Part print with two shaded views. Sizes in mm from the minimum x, y, z corner. Round coordinates to 2 decimals unless told otherwise and drop trailing zeros. Loops run counter-clockwise (first coordinate to the right, second up) from the corner with the lowest first, then second, coordinate; pieces in that order, holes last. Notation, with made-up numbers: (85, 4.25) - (131, 4.25) arc R6 ccw to (131, 13.25) - close; hole circle Ø10 at (45.5, -26). An arc over 180 degrees is marked (long way). Use a Markdown table: item, result.
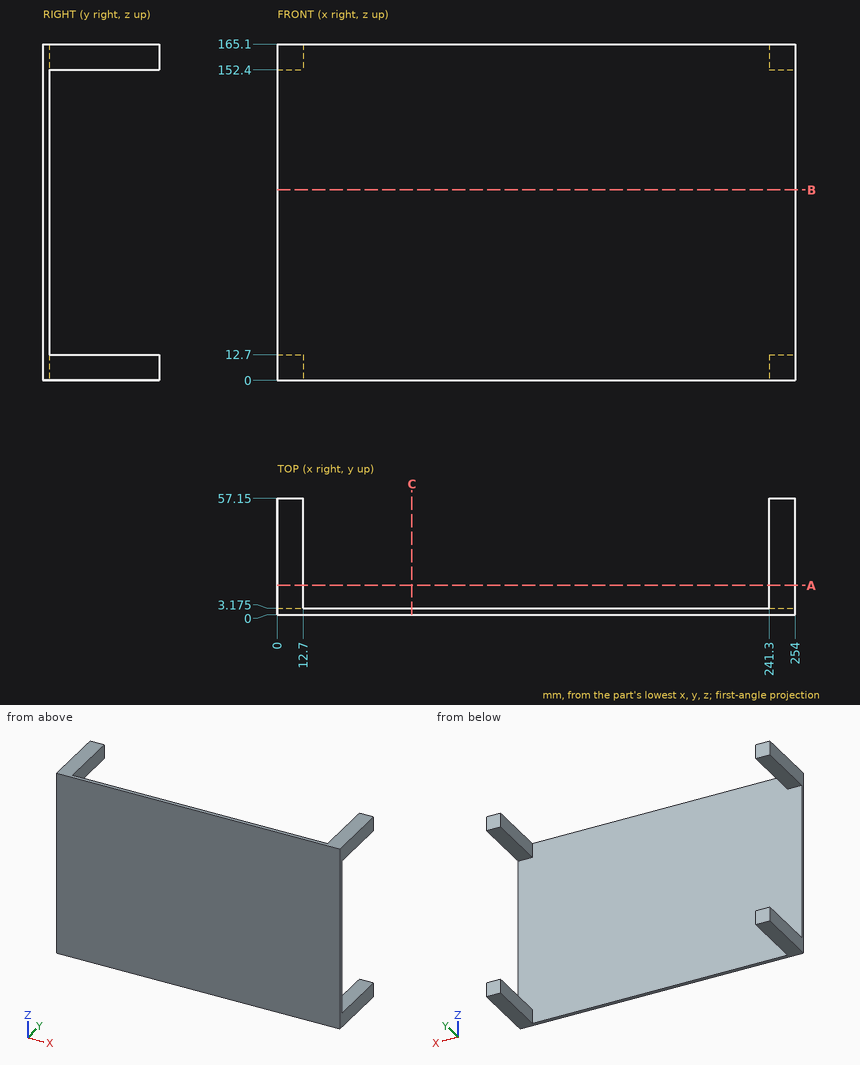
Q1. Probe line 1 (Z direction, x = 12, y = 49.5); line 2 (Y direction, x = 122.5, z = 90) (3 decimals). List the from-to ranges inside material, lowest first.
Results found:
| item | result |
|---|---|
| line 1 | z = 0 to 12.7, 152.4 to 165.1 |
| line 2 | y = 0 to 3.175 |
Q2. Cut at C-C, the plane x = 66. List the corners of the cut face in (y, z) (3 decimals), plus the area to 3 significant figures.
Results found:
| item | result |
|---|---|
| outline | (0, 0) - (3.175, 0) - (3.175, 165.1) - (0, 165.1) - close |
| area | 524 mm2 |
Q3. Cut at A-A, the plane y = 14.5. List the corners of the cut face in (x, z).
Results found:
| item | result |
|---|---|
| outline | (0, 0) - (12.7, 0) - (12.7, 12.7) - (0, 12.7) - close; (0, 152.4) - (12.7, 152.4) - (12.7, 165.1) - (0, 165.1) - close; (241.3, 0) - (254, 0) - (254, 12.7) - (241.3, 12.7) - close; (241.3, 152.4) - (254, 152.4) - (254, 165.1) - (241.3, 165.1) - close |
Q4. Drop flat-ended pins along their axis: pin 1 (5 mm diameter, centred on x = 53, z = 80, fed in from +Y) (3 decimals); pin 2 (12 mm diameter, centred on y = 47, z = 24.5, fed in from +X). Give the stop position or say it passes through.
Results found:
| item | result |
|---|---|
| pin 1 | stops at y = 3.175 |
| pin 2 | passes through |
Q5. Cut at B-B, the plane z = 93.5. List the corners of the cut face in (x, y) (3 decimals), plus the area to 3 significant figures.
Results found:
| item | result |
|---|---|
| outline | (0, 0) - (254, 0) - (254, 3.175) - (0, 3.175) - close |
| area | 806 mm2 |
